Check sheet for the modelled part. Datum: model origin and axes. Units: mm. A direction names the side the tool comes from. Coordinates: 2 decimals unless noted, no trailing zeros. Loops run counter-clockwise (first coordinate to the right, second up) from the corner with the lowest first, then second, coordinate; pieces in that order, holes last. Notation, with made-up numbers: M 1.5,64 L 23.5,64 A22 cw 23.5,96 Z; hole C 85.5,48 d4. An arc over 180 degrees is marked long. Return JSON: item names as keys, results as strings.
from build123d import *
from build123d.topology import SkipClean

# Parameters (mm, degrees)
BOSS_EXTRUDE1_DEPTH     = 3.5
CUT_EXTRUDE1_DEPTH      = 43.449971699
CUT_EXTRUDE1_DEPTH_BACK = 43.449971699
SKETCH3_R               = 2.75
SKETCH4_R               = 12.1
CUT_EXTRUDE2_DEPTH      = 5.1
BOSS_EXTRUDE2_START     = 0.5
SKETCH5_R               = 4.25
SKETCH5_R_2             = 2.75
BOSS_EXTRUDE2_DEPTH     = 0.5
SKETCH6_R               = 4.75
CUT_EXTRUDE3_DEPTH      = 4.5
FILLET1_R               = 5
CUT_EXTRUDE4_DEPTH      = 3.5


with BuildPart() as part:
    # Sketch1 → Boss-Extrude1 (new, symmetric)
    with BuildSketch(Plane.XY):
        with BuildLine():
            Line((32.00000152, 7.999997932), (32.00000152, -20))
            ThreePointArc((32.00000152, -20), (26.918315181, -26.732018471), (19.051409321, -23.689749429))
            Line((19.051409321, -23.689749429), (16.171450613, -19.04669704))
            ThreePointArc((16.171450613, -19.04669704), (12.060484849, -15.849407252), (6.85857128, -16.1))
            ThreePointArc((6.85857128, -16.1), (3.5, -17.146428199), (0, -17.5))
            Line((0, -17.5), (0, -11.6))
            ThreePointArc((0, -11.6), (11.6, 0), (0, 11.6))
            Line((0, 11.6), (0, 17))
            ThreePointArc((0, 17), (4.123105626, 16.492422502), (8, 15))
            Line((8, 15), (25.00000152, 15))
            ThreePointArc((25.00000152, 15), (29.949750451, 12.949746862), (32.00000152, 7.999997932))
        make_face()
    extrude(amount=BOSS_EXTRUDE1_DEPTH, both=True)

    # Sketch3 → Cut-Extrude1 (cut, two sides: drawn at the far end of the back side and taken through both)
    with BuildSketch(Plane.XY.offset(3.5).offset(-CUT_EXTRUDE1_DEPTH_BACK)):
        with Locations((25.00000152, 7.999998966)):
            Circle(SKETCH3_R)
        with Locations((25.00000152, -8.000001034)):
            Circle(SKETCH3_R)
        with Locations((25.00000152, -20.000001034)):
            Circle(SKETCH3_R)
    extrude(amount=CUT_EXTRUDE1_DEPTH + CUT_EXTRUDE1_DEPTH_BACK, mode=Mode.SUBTRACT)

    # Sketch4 → Cut-Extrude2 (cut)
    with BuildSketch(Plane(origin=(0, 0, -3.5), x_dir=(-1, 0, 0), z_dir=(0, 0, -1))):
        Circle(SKETCH4_R)
    extrude(amount=-CUT_EXTRUDE2_DEPTH, mode=Mode.SUBTRACT)

    # Sketch5 → Boss-Extrude2 (add)
    with BuildSketch(Plane.XY.offset(3.5).offset(BOSS_EXTRUDE2_START)):
        with Locations((25.00000152, -20.000001034)):
            Circle(SKETCH5_R)
        with Locations((25.00000152, -20.000001034)):
            Circle(SKETCH5_R_2, mode=Mode.SUBTRACT)
    extrude(amount=-BOSS_EXTRUDE2_DEPTH)

    # Sketch6 → Cut-Extrude3 (cut)
    with BuildSketch(Plane.XY.offset(3.5)):
        with Locations((25.00000152, -8.000001034)):
            Circle(SKETCH6_R)
        with Locations((25.00000152, 7.999998966)):
            Circle(SKETCH6_R)
    extrude(amount=-CUT_EXTRUDE3_DEPTH, mode=Mode.SUBTRACT)

    # Fillet1
    fillet1_edges = [part.edges().sort_by_distance(p)[0] for p in [
        (8, 15, 0),
    ]]
    fillet(fillet1_edges, radius=FILLET1_R)

    # Sketch8 → Cut-Extrude4 (cut)
    with BuildSketch(Plane(origin=(0, 0, -3.5), x_dir=(-1, 0, 0), z_dir=(0, 0, -1))):
        Polygon((-22.546262876, -15.750001034), (-27.453740164, -15.750001034), (-29.907478808, -20.000001034), (-27.453740164, -24.250001034), (-22.546262876, -24.250001034), (-20.092524232, -20.000001034), align=None)
    extrude(amount=-CUT_EXTRUDE4_DEPTH, mode=Mode.SUBTRACT)

    # Mirror2: part across plane


with BuildPart() as part_1:
    with SkipClean():  # the faces are left unmerged after this step: merging them gives an invalid solid
        add(part.part)
        add(part.part.mirror(Plane(origin=(0, 17, 3.5), x_dir=(0, 0, 1), z_dir=(1, 0, 0))))


solid = part_1.part
1) Go/stop test with flat-tipped pins: pin 1 Ø3 at (x, z) = (-2.5, -2) entering from +Y; pin 2 Ø7.5 at (x, y) = (-23, -9) entering from +Z; pin 3 Ø3 at (x, z) = (8.5, 1) entering from +Y. Record where each tip stops, or that it passes through.
Answers:
{"pin 1": "y = 16.97", "pin 2": "z = 3.5", "pin 3": "y = 15.49"}
2) Scan lines: line 1 along Y through (x, z) = (-25.5, 2.5); line 2 along X through (y, z) = (-19, 2.25); line 3 along X through (y, z) = (-21, 2). Record each from-to range of solid material in increasing order. Write a range as [from, to].
Answers:
{"line 1": "[-26.98, -22.7], [-17.3, -12.72], [-3.28, 3.28], [12.72, 14.98]", "line 2": "[-32, -27.56], [-22.44, -16.14], [16.14, 22.44], [27.56, 32]", "line 3": "[-31.93, -27.56], [-22.44, -17.38], [17.38, 22.44], [27.56, 31.93]"}
3) Section check B-B on z = 2.25. Record the cut outline in (x, y).
Answers:
{"outline": "M -32,-20 A7 ccw -19.05,-23.69 L -16.17,-19.05 A7.5 cw -6.86,-16.1 A17.5 ccw 6.86,-16.1 A7.5 cw 16.17,-19.05 L 19.05,-23.69 A7 ccw 32,-20 L 32,8 A7 ccw 25,15 L 9.17,15 A5 cw 7.08,15.45 A17 ccw -7.08,15.45 A5 cw -9.17,15 L -25,15 A7 ccw -32,8 Z; hole C -25,-8 d9.5; hole C -25,8 d9.5; hole C -25,-20 d5.5; hole C 0,0 d23.2; hole C 25,-8 d9.5; hole C 25,8 d9.5; hole C 25,-20 d5.5"}
4) Section check D-D on x = 13.5. Record the cut outline in (y, z), then the cut area to 3 significant figures.
Answers:
{"outline": "M -16.48,-3.5 L 15,-3.5 L 15,3.5 L -16.48,3.5 Z", "area": "220 mm²"}
5) Section check C-C on x = 3.5. Record the cut outline in (y, z).
Answers:
{"outline": "M -17.15,-3.5 L -11.58,-3.5 L -11.58,1.6 L -11.06,1.6 L -11.06,3.5 L -17.15,3.5 Z; M 11.06,1.6 L 11.58,1.6 L 11.58,-3.5 L 16.64,-3.5 L 16.64,3.5 L 11.06,3.5 Z"}
6) Set-up check for faces 1 (the face through (-17.63, -21.4, 0.05)), 2 (the face through (-28, -20, 4)), 3 (the face through (-24.642, -17.273, 2.028)), 4 (the face through (-21.337, -22.155, -1.774)), 5 (the face through (-28, -8, -1)): record each of +Z, -Z, +X, -X, +Y, -Y from which the full face is reachable in a straight line by a thin tool's end or side.
Answers:
{"face 1": "+Z, -Z, -Y", "face 2": "+Z, +X, -X, +Y, -Y", "face 3": "+Z, -Z", "face 4": "-Z", "face 5": "+Z"}
7) Section check A-A on y = 0. Record the cut outline in (x, z).
Answers:
{"outline": "M -32,-3.5 L -12.1,-3.5 L -12.1,1.6 L -11.6,1.6 L -11.6,3.5 L -32,3.5 Z; M 11.6,1.6 L 12.1,1.6 L 12.1,-3.5 L 32,-3.5 L 32,3.5 L 11.6,3.5 Z"}
8) Draft check along Y on faces 6 (the face through (22.973, 9.859, -2.267)), 7 (the face through (21.337, -22.155, -1.774)), 8 (the face through (-28.926, -21.628, 3.754)), 9 (the face through (17.63, -21.4, 0.05)). Enter one of: +Y half, -Y half, draft (parallel to the pull), parting line (faces both ways), or undercut.
Answers:
{"face 6": "undercut", "face 7": "undercut", "face 8": "parting line", "face 9": "-Y half"}
